The listing builds one solid part. Answer for the finished solid, in the listing's coordinates (mm). Round coordinates to 2 decimals unless told otherwise and drop trailing zeros. Write each loop counter-clockwise with the first axis right and the second up, starting at its lowest first coordinate (ties: lowest second). Pieces come first, ordered by that corner, then holes. Notation, with made-up numbers: (52, 58.5) - (97, 58.5) arc R14 ccw to (97, 74.5) - close; hole circle Ø4 at (16.25, 21). An arc over 180 degrees is marked (long way). Use a Markdown table: item, result. Add a question column.
1) Find the intervals of material crossed by probe 1 along Y at (x, z) = (-3.25, 1.75); probe 2 along X at (y, z) = (4.5, 4.15); probe 3 along X at (y, z) = (-1.75, 1.45), in increasing order. Write a range as from..to.
2) Each of these flat-tipped pins is pushed along its axis until it touches: P1, Ø2, axis at x = -1.5, y = -9, coming from the -Z side; P2, Ø12, axis at x = -7, y = 2.5, coming from the -Z side; P3, Ø13.5, axis at x = 0, y = 0, coming from the -Z side. Where does it stop, or does it pass through?
3) Determine the mould class of faces 1 (the cylindrical face through (-2.948, -13.277, 0.986)), 2 (the cylindrical face through (2.4, -4.5, 4.5)) for opening direction X: +X half, -X half, draft (parallel to the pull), parting line (faces both ways), or undercut.
4) A cutting plane is placed at A-A (z = 4). Give the vertices of the cut face in (x, y), then the cut area to 3 significant figures.
```python
from build123d import *


with BuildPart() as part:
    # Sketch → Revolve (revolve)
    with BuildSketch(Plane.XZ):
        with BuildLine():
            Line((5.1, 5.6), (5.1, 3.5))
            Line((5.271141, 3.328858), (5.1, 3.5))
            ThreePointArc((7.089877, 0.227339), (6.601658, 2.025061), (5.271141, 3.328858))
            Line((13.6, 0), (7.089877, 0.227339))
            Line((13.6, 2), (13.6, 0))
            Line((13.6, 2), (11.697984, 2.50964))
            ThreePointArc((9.520018, 4.886473), (10.262609, 3.380647), (11.697984, 2.50964))
            Line((9.5, 5), (9.520018, 4.886473))
            Line((9.5, 5), (6.52372, 5.260391))
            ThreePointArc((5.1, 5.6), (5.799366, 5.377817), (6.52372, 5.260391))
        make_face()
    revolve(axis=Axis((0, 0, 0), (0, 0, 1)))


solid = part.part
```
Entries:
| question | item | result |
|---|---|---|
| 1 | probe 1 | y = -13.21..-5.91, 5.91..13.21 |
| 1 | probe 2 | x = -8.65..-2.4, 2.4..8.65 |
| 1 | probe 3 | x = -13.49..-6.65, 6.65..13.49 |
| 2 | P1 | stops at z = 0.12 |
| 2 | P2 | stops at z = 0.01 |
| 2 | P3 | stops at z = 1.74 |
| 3 | face 1 | parting line |
| 3 | face 2 | undercut |
| 4 | outline | circle Ø19.65 at (0, 0); hole circle Ø10.2 at (0, 0) |
| 4 | area | 222 mm² |
